from build123d import *

# Parameters (mm, degrees)
SALIENTE_EXTRUIR1_DEPTH = 5.1


with BuildPart() as part:
    # Croquis1 → Saliente-Extruir1 (new body)
    with BuildSketch(Plane(origin=(0, 0, 0), x_dir=(1, 0, 0), z_dir=(0, 1, 0))):
        with BuildLine():
            Line((0, 0), (0, 6.8))
            Line((0, 6.8), (-8.8, 6.8))
            Line((-8.8, 6.8), (-8.8, 11.6))
            Line((-8.8, 11.6), (0, 11.6))
            Line((0, 11.6), (0, 18.4))
            Line((0, 18.4), (-8.8, 18.4))
            ThreePointArc((-8.8, 18.4), (-25.4, 35), (-8.8, 51.6))
            Line((-8.8, 51.6), (0, 51.6))
            Line((0, 51.6), (0, 58.4))
            Line((0, 58.4), (-8.8, 58.4))
            Line((-8.8, 58.4), (-8.8, 63.2))
            Line((-8.8, 63.2), (0, 63.2))
            Line((0, 63.2), (0, 70))
            Line((0, 70), (-8.8, 70))
            ThreePointArc((-8.8, 70), (-32.605724102, 60.57158363), (-43.5, 37.4))
            Line((-43.5, 37.4), (-34.7, 37.4))
            Line((-34.7, 37.4), (-34.7, 32.6))
            Line((-34.7, 32.6), (-43.5, 32.6))
            ThreePointArc((-43.5, 32.6), (-32.605724102, 9.42841637), (-8.8, 0))
            Line((-8.8, 0), (0, 0))
        make_face()
    extrude(amount=SALIENTE_EXTRUIR1_DEPTH)


solid = part.part
Verification items for the finished model (mm, model axes). A direction names the side the tool comes from. Round coordinates to 2 decimals unless told otherwise and drop trailing zeros. Loops run counter-clockwise (first coordinate to the right, second up) from the corner with the lowest first, then second, coordinate; pieces in that order, holes last. Notation, with made-up numbers: (84, 69.25) - (143, 69.25) arc R31 cw to (143, 106.25) - close; hole circle Ø5 at (-19, 8.25). An arc over 180 degrees is marked (long way). Use a Markdown table: item, result. Add a question column.
1. Release check for a two-part mould opening along Z. For faces 4 (the face through (-4, 3, -18.4)), 5 (the face through (0, 3, -67)), 6 (the face through (-4, 3, 0)) record: released by +Z, released by -Z, zero draft, split by the parting line, or undercut.
2. Section check A-A, the plane y = 2.85. Record the boundary of the cut face in (x, z).
3. Gauge pin test, flat ends, axial feed: pin 1 (1.5 mm diameter, centred on x = -5, y = 3.5, fed in from +Z); pin 2 (1.5 mm diameter, centred on y = 2, z = -46.5, fed in from +X); pin 3 (2.5 mm diameter, centred on x = -37, y = 3.5, fed in from +Z); pin 4 (1 mm diameter, centred on x = -10.5, y = 3.5, fed in from -Z). Record the tip position at first contact, or that the pin passes through.
4. Access from +Z, -Z, +X, -X, +Y, -Y to the whole of each face (thin tool, end or side, straight path). Record for faces 1 (the face through (-39, 3, -37.4)), 2 (the face through (-4, 3, -6.8)), 3 (the face through (-32.87, 2.51, -9.68)).
5. Thickness scan on probe 1 along Z at (x, y) = (-6.5, 1.6); probe 2 along Z at (x, y) = (-17, 3.75); probe 3 along Z at (x, y) = (-13.5, 0.35). Record the ranges inside material, lowest first. Write a range as [from, to].
6. Section check B-B, the plane z = -35. Record the boundary of the cut face in (x, y).
7. Section check C-C, the plane x = -33. Record the boundary of the cut face in (y, z).
Checks:
| question | item | result |
|---|---|---|
| 1 | face 4 | undercut |
| 1 | face 5 | zero draft |
| 1 | face 6 | released by +Z |
| 2 | outline | (-43.5, -37.4) arc R34.77 ccw to (-8.8, -70) - (0, -70) - (0, -63.2) - (-8.8, -63.2) - (-8.8, -58.4) - (0, -58.4) - (0, -51.6) - (-8.8, -51.6) arc R16.6 cw to (-8.8, -18.4) - (0, -18.4) - (0, -11.6) - (-8.8, -11.6) - (-8.8, -6.8) - (0, -6.8) - (0, 0) - (-8.8, 0) arc R34.77 ccw to (-43.5, -32.6) - (-34.7, -32.6) - (-34.7, -37.4) - close |
| 3 | pin 1 | stops at z = 0 |
| 3 | pin 2 | stops at x = -20 |
| 3 | pin 3 | stops at z = -12.8 |
| 3 | pin 4 | stops at z = -69.98 |
| 4 | face 1 | -X, +Y, -Y |
| 4 | face 2 | +X, +Y, -Y |
| 4 | face 3 | +Z, -X, +Y, -Y |
| 5 | probe 1 | z = [-70, -63.2], [-58.4, -51.6], [-18.4, -11.6], [-6.8, 0] |
| 5 | probe 2 | z = [-69.02, -49.43], [-20.57, -0.98] |
| 5 | probe 3 | z = [-69.68, -50.92], [-19.08, -0.32] |
| 6 | outline | (-34.7, 0) - (-25.4, 0) - (-25.4, 5.1) - (-34.7, 5.1) - close |
| 7 | outline | (0, -60.2) - (5.1, -60.2) - (5.1, -9.8) - (0, -9.8) - close |
